from build123d import *

# Parameters (mm, degrees)
F1_DEPTH = 600
F3_DEPTH = 600


with BuildPart() as f1:
    # F0 (on Front) → F1 (new body)
    with BuildSketch(Plane.XZ):
        Polygon((0, 80), (0, 0), (4, -4), (8, 0), (27, 0), (27.5, 0.5), (28, 0), (55, 0), (55, 19), (54.5, 19.5), (55, 20), (55, 60), (54.5, 60.5), (55, 61), (55, 80), (28, 80), (27.5, 79.5), (27, 80), (8, 80), (4, 84), align=None)
    extrude(amount=F1_DEPTH)

    # F2 (on Front) → F3 (cut, through all)
    with BuildSketch(Plane.XZ):
        with BuildLine():
            Line((5, 12), (9.398414, 12))
            Line((9.398414, 12), (8.156498, 9.912263))
            ThreePointArc((8.156498, 9.912263), (5.732233, 5.732233), (9.912263, 8.156498))
            Line((9.912263, 8.156498), (12, 9.398414))
            Line((12, 9.398414), (12, 5))
            Line((12, 5), (43, 5))
            Line((43, 5), (43, 9.398414))
            Line((43, 9.398414), (45.087737, 8.156498))
            ThreePointArc((45.087737, 8.156498), (49.267767, 5.732233), (46.843502, 9.912263))
            Line((46.843502, 9.912263), (45.601586, 12))
            Line((45.601586, 12), (50, 12))
            Line((50, 12), (50, 68))
            Line((50, 68), (45.601586, 68))
            Line((45.601586, 68), (46.230309, 70.346425))
            ThreePointArc((46.230309, 70.346425), (49.267767, 74.267767), (45.346425, 71.230309))
            Line((45.346425, 71.230309), (43, 70.601586))
            Line((43, 70.601586), (43, 75))
            Line((43, 75), (12, 75))
            Line((12, 75), (12, 70.601586))
            Line((12, 70.601586), (9.653575, 71.230309))
            ThreePointArc((9.653575, 71.230309), (5.732233, 74.267767), (8.769691, 70.346425))
            Line((8.769691, 70.346425), (9.398414, 68))
            Line((9.398414, 68), (5, 68))
            Line((5, 68), (5, 12))
        make_face()
    extrude(amount=F3_DEPTH, mode=Mode.SUBTRACT)


solid = f1.part
Input: part model. Units: mm. Frame: model coordinates. A direction names the side the tool comes from. Give positions to 0.01 mm unless a question says otherwise; leave off trailing zeros. Order: outer loops, then holes, each group sorted by start corner. A loop starts at its lowest first (then second) coordinate and runs counter-clockwise, first axis right, second up. Notation, with made-up numbers: (49.25, -8) - (95.25, -8) arc R18 ccw to (95.25, 27) - close; hole circle Ø2 at (40.5, 82.25). An arc over 180 degrees is marked (long way). Write each question's results on one line, items separated by ' | '.
Item 1: Draft query along Z for faces 1 (the flat face through (18, -296, 80)), 2 (the flat face through (3, 0, 41)), 3 (the flat face through (50, -296, 40)). Return one class per face: released by +Z, released by -Z, zero draft, split by the parting line, or undercut.
A:
face 1: released by +Z | face 2: zero draft | face 3: undercut
Item 2: Contact query for flat-ended pins moving along their axis: pin 1 Ø10 at (x, y) = (35.5, -452) entering from +Z; pin 2 Ø2 at (x, y) = (7.5, -386) entering from +Z; pin 3 Ø4 at (x, z) = (7.5, 72.5) entering from -Y; pin 4 Ø5 at (x, y) = (48, -229) entering from -Z. Output: stop coordinate, or through.
A:
pin 1: stops at z = 80 | pin 2: stops at z = 81.5 | pin 3: passes through | pin 4: stops at z = 0
Item 3: Section A-A (z = 54.5). Return loops of the section in (x, y).
A:
outline: (0, -600) - (5, -600) - (5, 0) - (0, 0) - close; (50, -600) - (55, -600) - (55, 0) - (50, 0) - close
Item 4: Access query for faces 4 (the flat face through (5, -296, 40)), 5 (the flat face through (17, -296, 0)), 6 (the flat face through (42, -296, 80)). Directions: +Z, -Z, +X, -X, +Y, -Y. A direction counts if a zero-diameter tool reaches every point of the face in a straight line with its end or side. Return the directions, or none.
A:
face 4: +Y, -Y | face 5: -Z, +X, +Y, -Y | face 6: +Z, +X, +Y, -Y
Item 5: Material intervals for line 1 along Z through (x, y) = (48, -65); line 2 along Z through (x, y) = (47.5, -270); line 3 along X through (y, z) = (-433.5, 7.5), sorted ascending.
A:
line 1: z = 0 to 5.05, 9.95 to 12, 68 to 70.05, 74.95 to 80 | line 2: z = 0 to 5, 10 to 12, 68 to 70, 75 to 80 | line 3: x = 0 to 5, 10 to 12, 43 to 45, 50 to 55
